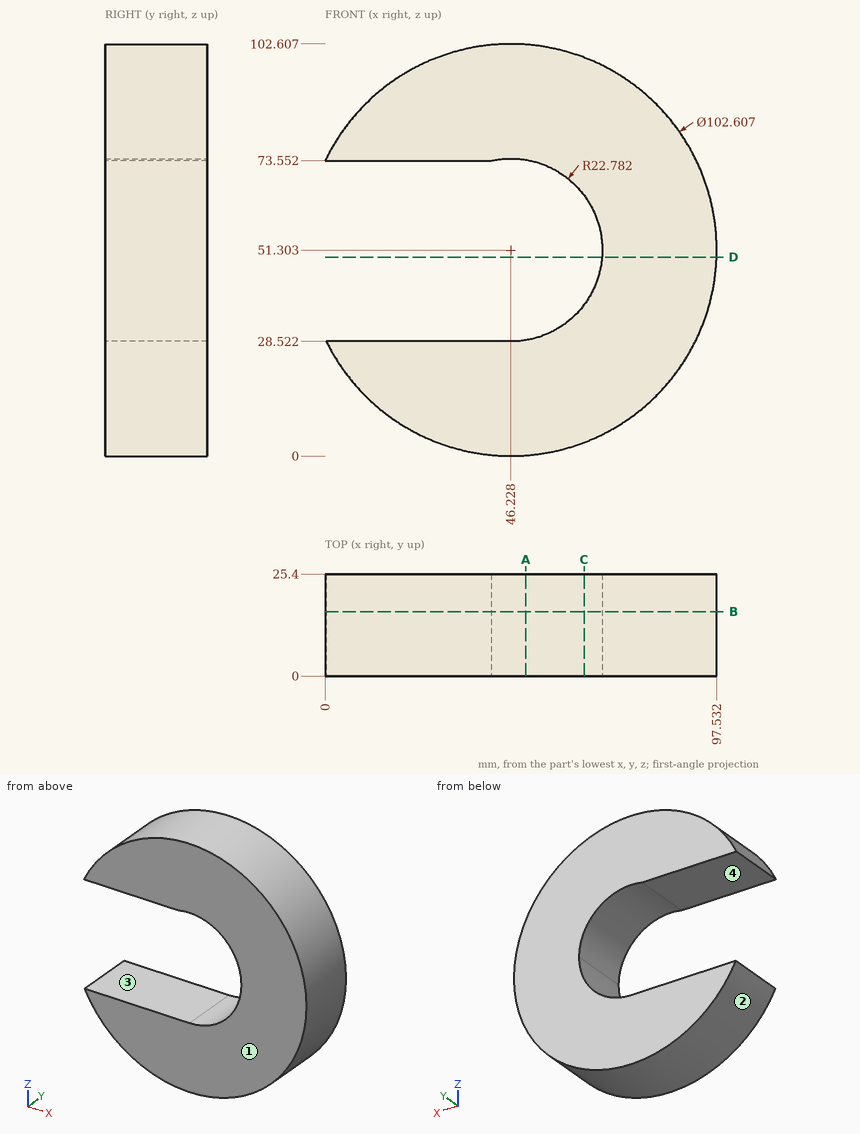
Here's the drawing with two shaded views (mm, measured from the low corner). I have some questions. Coordinates: 2 decimals unless noted, no trailing zeros. Loops run counter-clockwise (first coordinate to the right, second up) from the corner with the lowest first, then second, coordinate; pieces in that order, holes last. Notation, with made-up numbers: (50.25, -17) -> (75.25, -17) arc R23 ccw to (75.25, -7) -> close; hole circle Ø11 at (20, 19). An arc over 180 degrees is marked (long way). Answer in a Markdown table with one row per item.
(1) Will these pins go through, and if not, where does the flat tip stop? pin 1 Ø1 at (y, z) = (16.5, 43.5) entering from +X; pin 2 Ø6 at (x, z) = (43, 69.5) entering from -Y; pin 3 Ø3 at (y, z) = (17, 48) entering from +X; pin 4 Ø5 at (x, y) = (59.5, 15.5) entering from -Z.
Results found:
| item | result |
|---|---|
| pin 1 | stops at x = 97.01 |
| pin 2 | passes through |
| pin 3 | stops at x = 97.5 |
| pin 4 | stops at z = 1.14 |
(2) Imagine slicing it at D-D (z = 49.5). List the corners of the cut face in (x, y) for me.
Results found:
| item | result |
|---|---|
| outline | (68.94, 0) -> (97.5, 0) -> (97.5, 25.4) -> (68.94, 25.4) -> close |
(3) Imagine slicing it at B-B (y = 16). List the corners of the cut face in (x, z) for me, plus the area to 3 significant figures.
Results found:
| item | result |
|---|---|
| outline | (0, 73.55) -> (41.33, 73.55) arc R22.78 cw (long way) to (46.23, 28.52) -> (0.26, 28.52) arc R51.3 ccw (long way) to start |
| area | 5,220 mm^2 |
(4) Imagine slicing it at C-C (x = 64.5). List the corners of the cut face in (y, z) for me (1 decimal), plus the area to 3 significant figures.
Results found:
| item | result |
|---|---|
| outline | (0, 3.4) -> (25.4, 3.4) -> (25.4, 37.7) -> (0, 37.7) -> close; (0, 64.9) -> (25.4, 64.9) -> (25.4, 99.2) -> (0, 99.2) -> close |
| area | 1,740 mm^2 |
(5) If I drill on probe 1 along Z at (x, y) = (35.5, 16.5) (1 decimal); probe 2 along X at (y, z) = (21, 89.5) (1 decimal); probe 3 along X at (y, z) = (2.5, 13) (1 decimal), over which ranges is the centre line in solid material (lowest first)?
Results found:
| item | result |
|---|---|
| probe 1 | z = 1.1 to 28.5, 73.6 to 101.5 |
| probe 2 | x = 12 to 80.5 |
| probe 3 | x = 12.1 to 80.4 |
(6) Imagine slicing it at A-A (x = 50). List the corners of the cut face in (y, z) for me.
Results found:
| item | result |
|---|---|
| outline | (0, 0.14) -> (25.4, 0.14) -> (25.4, 28.84) -> (0, 28.84) -> close; (0, 73.77) -> (25.4, 73.77) -> (25.4, 102.47) -> (0, 102.47) -> close |
(7) Thinking about a two-plate mould opening in Z: for the marked faces 1, 2, 3 and 4, which applies, released by +Z, released by -Z, zero draft, split by the parting line, or undercut?
Results found:
| item | result |
|---|---|
| face 1 | zero draft |
| face 2 | split by the parting line |
| face 3 | undercut |
| face 4 | undercut |
